Here's how the part is built. I have some questions about the finished solid (model axes, mm). A direction names the side the tool comes from. Round coordinates to 2 decimals unless told otherwise and drop trailing zeros. Loops run counter-clockwise (first coordinate to the right, second up) from the corner with the lowest first, then second, coordinate; pieces in that order, holes last. Notation, with made-up numbers: M 68,46.5 L 90,46.5 A17 cw 90,65.5 Z; hole C 85.5,-9 d4. An arc over 180 degrees is marked long. Put each result on its own line as item: value. Start each with the question number.
```python
from build123d import *

# Parameters (mm, degrees)
SKETCH_1_R          = 10
EXTRUDE_1_DEPTH     = 22
SKETCH_4_W          = 3.52564581
SKETCH_4_H          = 12
CUT_EXTRUDE_1_DEPTH = 22
FILLET_1_R          = 1
SKETCH2_W           = 5.25
SKETCH2_H           = 19


with BuildPart() as part:
    # ｽｹｯﾁ1 → ﾎﾞｽ - 押し出し1 (new, symmetric)
    with BuildSketch(Plane(origin=(0, 0, 0), x_dir=(1, 0, 0), z_dir=(0, 1, 0))):
        with Locations(Location((0, 0, 0), (0, 0, 270))):
            Circle(SKETCH_1_R)
    extrude(amount=EXTRUDE_1_DEPTH, both=True)

    # ｽｹｯﾁ4 → ｶｯﾄ - 押し出し1 (cut, symmetric)
    with BuildSketch(Plane(origin=(0, 0, 0), x_dir=(0, 0, -1), z_dir=(1, 0, 0))):
        with Locations((-10.762822905, 0)):
            Rectangle(SKETCH_4_W, SKETCH_4_H)
        with Locations((10.762822905, 0)):
            Rectangle(SKETCH_4_W, SKETCH_4_H)
    extrude(amount=CUT_EXTRUDE_1_DEPTH, both=True, mode=Mode.SUBTRACT)

    # ﾌｨﾚｯﾄ1
    fillet_1_edges = [part.edges().sort_by_distance(p)[0] for p in [
        (0, -6, -9),
        (0, 6, -9),
        (0, -6, 9),
        (0, 6, 9),
    ]]
    fillet(fillet_1_edges, radius=FILLET_1_R - 0.0001)  # a hair under: the kernel refuses the full size

    # Sketch2 → M12x1.5 ねじ穴1 (revolve, cut)
    with BuildSketch(Plane(origin=(0, 0, 9), x_dir=(0, -1, 0), z_dir=(1, 0, 0))):
        with Locations((2.625, 9.5)):
            Rectangle(SKETCH2_W, SKETCH2_H)
    revolve(axis=Axis((0, 0, 15.35), (0, 0, -1)), mode=Mode.SUBTRACT)


solid = part.part
```
1) Suppose I cut it at D-D (x = 2.5). Write out the boundary of the cut face in (y, z), plus the area to 3 significant figures.
2) On a 3-axis mill with a long thin cutter (end or side, diameter ignored), from which of +Z, -Z, +X, -X, +Y, -Y can I reach the whole of each face in a straight line? I mean faces 1 (the face through (-4, -4, 9)), 2 (the face through (4, -4, -9)), 3 (the face through (-6, 0, -8)), 4 (the face through (-1.6, -5, -0.1)). Say none if no direction works.
3) If we mould it in two halves opening along Y, with no side actions, what happens to faces 5 (the face through (0, 22, 0)), 6 (the face through (0.1, -5.6, -9.2)), 7 (the face through (0, -22, 0))? For each: pulls with the +Y half, pulls with the -Y half, needs draft (parallel to the pull), parting line crosses it, or undercut.
4) Suppose I cut it at B-B (z = 0). Write out the boundary of the cut face in (x, y).
5) Suppose I cut it at A-A (x = -1). Write out the boundary of the cut face in (y, z), plus the area to 3 significant figures.
6) I'm going to push flat-ended pins straight in: P1, Ø1.5, axis at x = -4.5, y = 16.5, coming from the +Z side; P2, Ø6, axis at x = -7.5, y = 3, coming from the +Z side; P3, Ø2.5, axis at x = -3, y = 4.5, coming from the -Z side; P4, Ø1.7, axis at x = 2.5, y = 3.5, coming from the +Z side. Where does each tip first touch, or does it pass through?
7) If I drill on probe 1 along Y at (x, z) = (0, 0.75); probe 2 along X at (y, z) = (0, 1.25); probe 3 along X at (y, z) = (0, 2.5), over which ranges is the centre line in solid material (lowest first)? Write a range as from..to.
8) Suppose I cut it at C-C (y = 0). Write out the boundary of the cut face in (x, z), plus the area to 3 significant figures.
Results are:
1. outline: M -22,-9.68 L -5.95,-9.68 A1 cw -5,-9 L -4.62,-9 L -4.62,9 L -5,9 A1 cw -5.95,9.68 L -22,9.68 Z; M 4.62,-9 L 5,-9 A1 cw 5.95,-9.68 L 22,-9.68 L 22,9.68 L 5.95,9.68 A1 cw 5,9 L 4.62,9 Z
1. area: 670 mm²
2. face 1: +Z, +X, -X
2. face 2: -Z, +X, -X
2. face 3: +Y, -Y
2. face 4: -Z
3. face 5: pulls with the +Y half
3. face 6: undercut
3. face 7: pulls with the -Y half
4. outline: M -10,-22 L 10,-22 L 10,22 L -10,22 Z; hole C 0,0 d10.5
5. outline: M -22,-9.95 L -6,-9.95 A1 cw -5.15,-9.01 L -5.15,9 L -5,9 A1 cw -6,9.95 L -22,9.95 Z; M 5,9 L 5.15,9 L 5.15,-9.01 A1 cw 6,-9.95 L 22,-9.95 L 22,9.95 L 6,9.95 A1 cw Z
5. area: 668 mm²
6. P1: z = 9.27
6. P2: z = 8.93
6. P3: z = -9.34
6. P4: through
7. probe 1: -22..-5.25, 5.25..22
7. probe 2: -9.92..-5.25, 5.25..9.92
7. probe 3: -9.68..-5.25, 5.25..9.68
8. outline: M -5.25,-8.51 L -5.25,8.51 A10 ccw Z; M 5.25,-8.51 A10 ccw 5.25,8.51 Z
8. area: 114 mm²
